Read the model definition and answer for the solid it produces. Units are mm, in the model's axes. Face numbers are marked on the shaded views. A direction names the side the tool comes from. Give positions to 0.01 mm unless a question says otherwise; leave off trailing zeros. Loops run counter-clockwise (first coordinate to the right, second up) from the corner with the lowest first, then second, coordinate; pieces in that order, holes last. Notation, with made-up numbers: (85, -30) -> (104, -30) arc R19 ccw to (104, -14) -> close; hole circle Ø9 at (50.25, 61). An arc over 180 degrees is marked (long way). Write each question's results on one line, items separated by ' | '. Start each with the question number.
Item 1: Find the intervals of material crossed by line 1 (Z direction, x = -58, y = -5.5); line 2 (Z direction, x = -9, y = 0.25); line 3 (Y direction, x = -4, z = 14.5), in increasing order.
Item 2: Each of these flat-tipped pins is pushed along its axis until it touches: P1, Ø1, axis at y = -5.5, z = -9.5, coming from the -X side; P2, Ø10, axis at x = -88, y = -9, coming from the +Z side; P3, Ø1, axis at y = -4.5, z = 21.5, coming from the -X side; P4, Ø8, axis at x = -65.5, z = 35.5, coming from the -Y side. Where does it stop, or does it pass through?
Item 3: Section A-A on y = -9 is taken. Write down the section's boundary in (x, z), and give its area (3 significant figures).
Item 4: Section D-D on x = -6.5 is taken. Write down the section's boundary in (y, z), and give its area (3 significant figures).
Item 5: Which of the six approach directions +Z, -Z, +X, -X, +Y, -Y give full straight-line access (tool end or side, diameter ignored) to the marked faces 1 and 2?
Item 6: Section B-B on x = -30 is taken. Write down the section's boundary in (y, z).
Item 7: Section C-C on z = -41 is taken. Write down the section's boundary in (x, y).
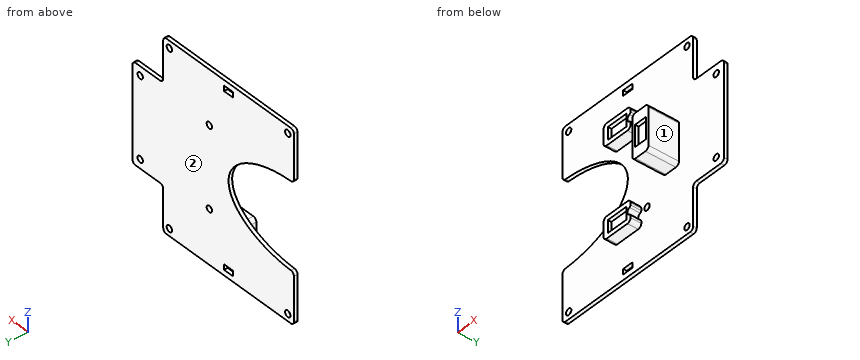
```python
from build123d import *

# Parameters (mm, degrees)
SKETCH1_R           = 1.75
SKETCH1_W           = 6
SKETCH1_H           = 3
BOSS_EXTRUDE1_DEPTH = 2
BOSS_EXTRUDE2_DEPTH = 6
SKETCH4_RX          = 42.5
SKETCH4_RY          = 24
CUT_EXTRUDE1_DEPTH  = 2
BOSS_EXTRUDE3_DEPTH = 17
FILLET1_R           = 2
CUT_EXTRUDE2_START  = -6
SKETCH2_3_W         = 12
SKETCH2_3_H         = 7
CUT_EXTRUDE2_DEPTH  = 2
CUT_EXTRUDE3_START  = -17
SKETCH3_3_W         = 7
SKETCH3_3_H         = 12
CUT_EXTRUDE3_DEPTH  = 2


with BuildPart() as part:
    # Sketch1 → Boss-Extrude1 (new body)
    with BuildSketch(Plane(origin=(0, 0, 0), x_dir=(1, 0, 0), z_dir=(0, 1, 0))):
        Polygon((-100.077357964, 56.197183099), (-15.077357964, 56.197183099), (-15.077357964, 31.197183099), (4.922642036, 31.197183099), (4.922642036, -23.802816901), (-15.077357964, -23.802816901), (-15.077357964, -48.802816901), (-100.077357964, -48.802816901), align=None)
        with Locations(Location((-96.077357964, 52.197183099, 0), (0, 0, 270))):  # turned: the seam where the file's is
            Circle(SKETCH1_R, mode=Mode.SUBTRACT)
        with Locations(Location((-96.077357964, -44.802816901, 0), (0, 0, 270))):  # turned: the seam where the file's is
            Circle(SKETCH1_R, mode=Mode.SUBTRACT)
        with Locations(Location((-19.077357964, -44.802816901, 0), (0, 0, 270))):  # turned: the seam where the file's is
            Circle(SKETCH1_R, mode=Mode.SUBTRACT)
        with Locations(Location((-19.077357964, 52.197183099, 0), (0, 0, 270))):  # turned: the seam where the file's is
            Circle(SKETCH1_R, mode=Mode.SUBTRACT)
        with Locations(Location((-0.077357964, 26.197183099, 0), (0, 0, 270))):  # turned: the seam where the file's is
            Circle(SKETCH1_R, mode=Mode.SUBTRACT)
        with Locations(Location((-0.077357964, -18.802816901, 0), (0, 0, 270))):  # turned: the seam where the file's is
            Circle(SKETCH1_R, mode=Mode.SUBTRACT)
        with Locations(Location((-45.077357964, 26.197183099, 0), (0, 0, 270))):  # turned: the seam where the file's is
            Circle(SKETCH1_R, mode=Mode.SUBTRACT)
        with Locations(Location((-45.077357964, -18.802816901, 0), (0, 0, 270))):  # turned: the seam where the file's is
            Circle(SKETCH1_R, mode=Mode.SUBTRACT)
        with Locations((-57.581758556, 51.697183099)):
            Rectangle(SKETCH1_W, SKETCH1_H, mode=Mode.SUBTRACT)
        with Locations((-57.577357964, -44.302816901)):
            Rectangle(SKETCH1_W, SKETCH1_H, mode=Mode.SUBTRACT)
    extrude(amount=BOSS_EXTRUDE1_DEPTH)

    # Sketch2 → Boss-Extrude2 (add)
    with BuildSketch(Plane(origin=(0, 0, 0), x_dir=(1, 0, 0), z_dir=(0, 1, 0))):
        with BuildLine():
            Line((-48.827357964, 32.697183099), (-48.827357964, 31.525610223))
            ThreePointArc((-48.827357964, 31.525610223), (-49.010861383, 30.948259954), (-49.494024631, 30.582801182))
            ThreePointArc((-49.494024631, 30.582801182), (-50.827357964, 28.697183099), (-49.494024631, 26.811565015))
            ThreePointArc((-49.494024631, 26.811565015), (-49.010861383, 26.446106243), (-48.827357964, 25.868755974))
            Line((-48.827357964, 25.868755974), (-48.827357964, 24.697183099))
            ThreePointArc((-48.827357964, 24.697183099), (-49.413144402, 23.282969536), (-50.827357964, 22.697183099))
            Line((-50.827357964, 22.697183099), (-64.327357964, 22.697183099))
            ThreePointArc((-64.327357964, 22.697183099), (-65.741571527, 23.282969536), (-66.327357964, 24.697183099))
            Line((-66.327357964, 24.697183099), (-66.327357964, 32.697183099))
            ThreePointArc((-66.327357964, 32.697183099), (-65.741571527, 34.111396661), (-64.327357964, 34.697183099))
            Line((-64.327357964, 34.697183099), (-50.827357964, 34.697183099))
            ThreePointArc((-50.827357964, 34.697183099), (-49.413144402, 34.111396661), (-48.827357964, 32.697183099))
        make_face()
        with BuildLine():
            Line((-48.822971012, -17.300189586), (-48.822971012, -18.471355074))
            ThreePointArc((-48.822971012, -18.471355074), (-49.00663465, -19.04893186), (-49.4901609, -19.414348939))
            ThreePointArc((-49.4901609, -19.414348939), (-50.8246687, -21.299453668), (-49.492167868, -23.185977571))
            ThreePointArc((-49.492167868, -23.185977571), (-49.009337779, -23.551474397), (-48.825981367, -24.128616711))
            Line((-48.825981367, -24.128616711), (-48.825981367, -25.300189586))
            ThreePointArc((-48.825981367, -25.300189586), (-49.411767805, -26.714403149), (-50.825981367, -27.300189586))
            Line((-50.825981367, -27.300189586), (-64.322971012, -27.300189586))
            ThreePointArc((-64.322971012, -27.300189586), (-65.737184574, -26.714403149), (-66.322971012, -25.300189586))
            Line((-66.322971012, -25.300189586), (-66.322971012, -17.300189586))
            ThreePointArc((-66.322971012, -17.300189586), (-65.737184574, -15.885976024), (-64.322971012, -15.300189586))
            Line((-64.322971012, -15.300189586), (-50.822971012, -15.300189586))
            ThreePointArc((-50.822971012, -15.300189586), (-49.408757449, -15.885976024), (-48.822971012, -17.300189586))
        make_face()
    extrude(amount=-BOSS_EXTRUDE2_DEPTH)

    # Sketch4 → Cut-Extrude1 (cut)
    with BuildSketch(Plane(origin=(0, 0, 0), x_dir=(1, 0, 0), z_dir=(0, 1, 0))):
        with Locations(Location((-100.077357964, 3.697183099), (0, 0, 0))):
            Ellipse(SKETCH4_RX, SKETCH4_RY)
    extrude(amount=CUT_EXTRUDE1_DEPTH, mode=Mode.SUBTRACT)

    # Sketch3 → Boss-Extrude3 (add)
    with BuildSketch(Plane(origin=(0, 0, 0), x_dir=(1, 0, 0), z_dir=(0, 1, 0))):
        with BuildLine():
            Line((-32.827357964, 15.947183099), (-26.327357964, 15.947183099))
            ThreePointArc((-26.327357964, 15.947183099), (-24.913144402, 15.361396661), (-24.327357964, 13.947183099))
            Line((-24.327357964, 13.947183099), (-24.327357964, -6.552816901))
            ThreePointArc((-24.327357964, -6.552816901), (-24.913144402, -7.967030464), (-26.327357964, -8.552816901))
            Line((-26.327357964, -8.552816901), (-32.827357964, -8.552816901))
            ThreePointArc((-32.827357964, -8.552816901), (-34.241571527, -7.967030464), (-34.827357964, -6.552816901))
            Line((-34.827357964, -6.552816901), (-34.827357964, 13.947183099))
            ThreePointArc((-34.827357964, 13.947183099), (-34.241571527, 15.361396661), (-32.827357964, 15.947183099))
        make_face()
    extrude(amount=-BOSS_EXTRUDE3_DEPTH)

    # Fillet1
    fillet1_edges = [part.edges().sort_by_distance(p)[0] for p in [
        (-100.077357964, 1, -56.197183099),
        (-100.077357964, 1, -27.697183099),
        (-100.077357964, 1, 20.302816901),
        (-100.077357964, 1, 48.802816901),
        (-15.077357964, 1, 48.802816901),
        (-15.077357964, 1, 23.802816901),
        (4.922642036, 1, 23.802816901),
        (4.922642036, 1, -31.197183099),
        (-15.077357964, 1, -31.197183099),
        (-15.077357964, 1, -56.197183099),
    ]]
    fillet(fillet1_edges, radius=FILLET1_R)

    # Sketch2_3 → Cut-Extrude2 (cut)
    with BuildSketch(Plane(origin=(0, 0, 0), x_dir=(1, 0, 0), z_dir=(0, 1, 0)).offset(CUT_EXTRUDE2_START)):
        with Locations((-57.577357964, 28.697183099)):
            Rectangle(SKETCH2_3_W, SKETCH2_3_H)
        with Locations((-57.574476189, -21.300189586)):
            Rectangle(SKETCH2_3_W, SKETCH2_3_H)
    extrude(amount=CUT_EXTRUDE2_DEPTH, mode=Mode.SUBTRACT)

    # Sketch3_3 → Cut-Extrude3 (cut)
    with BuildSketch(Plane(origin=(0, 0, 0), x_dir=(1, 0, 0), z_dir=(0, 1, 0)).offset(CUT_EXTRUDE3_START)):
        with Locations((-29.577357964, 3.697183099)):
            Rectangle(SKETCH3_3_W, SKETCH3_3_H)
    extrude(amount=CUT_EXTRUDE3_DEPTH, mode=Mode.SUBTRACT)


solid = part.part
```
Findings:
1) line 1: -34.7 to -32.2, -25.2 to -22.7, 15.3 to 17.8, 24.8 to 27.3 | line 2: -31.2 to 23.8 | line 3: 0 to 2
2) P1: x = -34.83 | P2: through | P3: x = -66.32 | P4: y = 0
3) outline: (-34.83, -13.95) arc R2 ccw to (-32.83, -15.95) -> (-26.33, -15.95) arc R2 ccw to (-24.33, -13.95) -> (-24.33, 6.55) arc R2 ccw to (-26.33, 8.55) -> (-32.83, 8.55) arc R2 ccw to (-34.83, 6.55) -> close | area: 254 mm2
4) outline: (0, -31.2) -> (2, -31.2) -> (2, 23.8) -> (0, 23.8) -> close | area: 110 mm2
5) face 1: +Z, -Z, +X, -Y | face 2: +Z, -Z, +X, -X, +Y
6) outline: (-17, -15.95) -> (0, -15.95) -> (0, -56.2) -> (2, -56.2) -> (2, 48.8) -> (0, 48.8) -> (0, 8.55) -> (-17, 8.55) -> (-17, 2.3) -> (-15, 2.3) -> (-15, -9.7) -> (-17, -9.7) -> close
7) outline: (-100.08, 0) -> (-15.08, 0) -> (-15.08, 2) -> (-100.08, 2) -> close
